from build123d import *

# Parameters (mm, degrees)
SKETCH1_R           = 32.5
SKETCH1_R_2         = 7.5
SKETCH1_W           = 5
SKETCH1_H           = 5
BOSS_EXTRUDE1_DEPTH = 3
SKETCH2_R           = 0.75
CUT_EXTRUDE1_DEPTH  = 47.059743812


with BuildPart() as part:
    # Sketch1 → Boss-Extrude1 (new body)
    with BuildSketch(Plane(origin=(0, 0, 0), x_dir=(1, 0, 0), z_dir=(0, 1, 0))):
        with Locations(Location((0, 0, 0), (0, 0, 270))):
            Circle(SKETCH1_R)
        with Locations(Location((0, 0, 0), (0, 0, 270))):
            Circle(SKETCH1_R_2, mode=Mode.SUBTRACT)
        with Locations((-13.5, -20)):
            Rectangle(SKETCH1_W, SKETCH1_H, mode=Mode.SUBTRACT)
        with Locations((-13.5, 20)):
            Rectangle(SKETCH1_W, SKETCH1_H, mode=Mode.SUBTRACT)
        with Locations((13.5, 20)):
            Rectangle(SKETCH1_W, SKETCH1_H, mode=Mode.SUBTRACT)
        with Locations((13.5, -20)):
            Rectangle(SKETCH1_W, SKETCH1_H, mode=Mode.SUBTRACT)
    extrude(amount=BOSS_EXTRUDE1_DEPTH)

    # Sketch2 → Cut-Extrude1 (cut, through all)
    with BuildSketch(Plane.XZ):
        with Locations(Location((0, -29.5, 0), (0, 0, 270))):
            Circle(SKETCH2_R)
        with Locations(Location((-9.116001334, -28.056167231, 0), (0, 0, 270))):
            Circle(SKETCH2_R)
        with Locations(Location((-17.339664943, -23.866001334, 0), (0, 0, 270))):
            Circle(SKETCH2_R)
        with Locations(Location((-23.866001334, -17.339664943, 0), (0, 0, 270))):
            Circle(SKETCH2_R)
        with Locations(Location((-28.056167231, -9.116001334, 0), (0, 0, 270))):
            Circle(SKETCH2_R)
        with Locations(Location((-29.5, 0, 0), (0, 0, 270))):
            Circle(SKETCH2_R)
        with Locations(Location((-28.056167231, 9.116001334, 0), (0, 0, 270))):
            Circle(SKETCH2_R)
        with Locations(Location((-23.866001334, 17.339664943, 0), (0, 0, 270))):
            Circle(SKETCH2_R)
        with Locations(Location((-17.339664943, 23.866001334, 0), (0, 0, 270))):
            Circle(SKETCH2_R)
        with Locations(Location((-9.116001334, 28.056167231, 0), (0, 0, 270))):
            Circle(SKETCH2_R)
        with Locations(Location((0, 29.5, 0), (0, 0, 270))):
            Circle(SKETCH2_R)
        with Locations(Location((9.116001334, 28.056167231, 0), (0, 0, 270))):
            Circle(SKETCH2_R)
        with Locations(Location((17.339664943, 23.866001334, 0), (0, 0, 270))):
            Circle(SKETCH2_R)
        with Locations(Location((23.866001334, 17.339664943, 0), (0, 0, 270))):
            Circle(SKETCH2_R)
        with Locations(Location((28.056167231, 9.116001334, 0), (0, 0, 270))):
            Circle(SKETCH2_R)
        with Locations(Location((29.5, 0, 0), (0, 0, 270))):
            Circle(SKETCH2_R)
        with Locations(Location((28.056167231, -9.116001334, 0), (0, 0, 270))):
            Circle(SKETCH2_R)
        with Locations(Location((23.866001334, -17.339664943, 0), (0, 0, 270))):
            Circle(SKETCH2_R)
        with Locations(Location((17.339664943, -23.866001334, 0), (0, 0, 270))):
            Circle(SKETCH2_R)
        with Locations(Location((9.116001334, -28.056167231, 0), (0, 0, 270))):
            Circle(SKETCH2_R)
    extrude(amount=-CUT_EXTRUDE1_DEPTH, mode=Mode.SUBTRACT)


solid = part.part
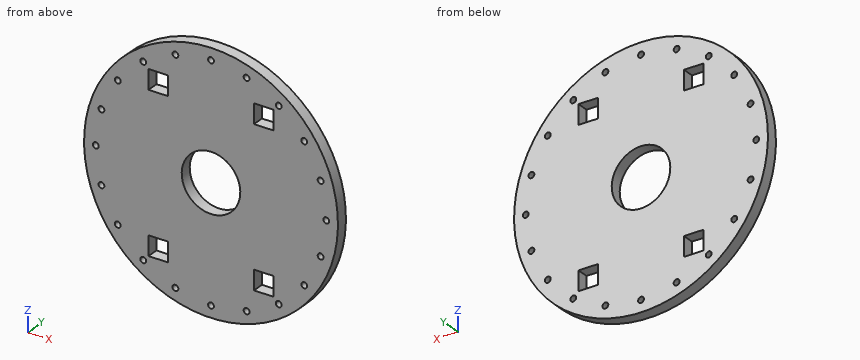
The model under review builds one solid part; all positions refer to its coordinate system, in mm. Round coordinates to 2 decimals unless told otherwise and drop trailing zeros. Write each loop counter-clockwise with the first axis right and the second up, starting at its lowest first coordinate (ties: lowest second). Pieces come first, ordered by that corner, then holes. Notation, with made-up numbers: M 77.5,25 L 106.5,25 A35 ccw 106.5,57 Z; hole C -27,-2 d9. An arc over 180 degrees is marked long. Answer as CSV lines item,"result". Start each with the question number.
Q1. Wall thickness on line 1 along X through (y, z) = (2.2, -19); line 2 along Z through (x, y) = (-12.5, 2.05); line 3 along X through (y, z) = (2.2, -24): over which ranges is each line inside the solid? List them lowest first.
Q2. Consider section B-B, the plane x = 0. Give the boundary of the cut face in (y, z).
Q3. Consider section C-C, the plane z = -19.5. Give the boundary of the cut face in (x, y).
Q4. Consider section D-D, the plane y = 0.9. State how many separate pieces and enclosed holes the cut face has, then the cut area to 3 significant figures.
Q5. Clearance check with a flat-ended pin moving along its axis: P1, Ø1.5, axis at y = 1, z = 19, coming from the +X side. State where the tip first meets the part, or that it passes through.
Q6. Consider section A-A, the plane z = 0. Give the boundary of the cut face in (x, y).
Result set:
1,line 1,"x = -26.37 to -16, -11 to 11, 16 to 26.37"
1,line 2,"z = -30 to -22.5, -17.5 to 17.5, 22.5 to 30"
1,line 3,"x = -21.91 to -18.08, -16.6 to 16.6, 18.08 to 21.91"
2,outline,"M 0,-32.5 L 3,-32.5 L 3,-30.25 L 0,-30.25 Z; M 0,-28.75 L 3,-28.75 L 3,-7.5 L 0,-7.5 Z; M 0,7.5 L 3,7.5 L 3,28.75 L 0,28.75 Z; M 0,30.25 L 3,30.25 L 3,32.5 L 0,32.5 Z"
3,outline,"M -26,0 L -16,0 L -16,3 L -26,3 Z; M -11,0 L 11,0 L 11,3 L -11,3 Z; M 16,0 L 26,0 L 26,3 L 16,3 Z"
4,separate pieces,"1"
4,enclosed holes,"25"
4,area,"3,010 mm²"
5,P1,"stops at x = 26.89"
6,outline,"M -32.5,0 L -30.25,0 L -30.25,3 L -32.5,3 Z; M -28.75,0 L -7.5,0 L -7.5,3 L -28.75,3 Z; M 7.5,0 L 28.75,0 L 28.75,3 L 7.5,3 Z; M 30.25,0 L 32.5,0 L 32.5,3 L 30.25,3 Z"
